```python
from build123d import *

# Parameters (mm, degrees)
SKETCH2_R           = 1.5
BOSS_EXTRUDE1_DEPTH = 2.54
SKETCH3_R           = 3.175
SKETCH3_R_2         = 1.5
BOSS_EXTRUDE2_DEPTH = 0.635
SKETCH4_W           = 6.35
SKETCH4_H           = 3
BOSS_EXTRUDE3_DEPTH = 3


with BuildPart() as part:
    # Sketch2 → Boss-Extrude1 (new body)
    with BuildSketch(Plane.XY):
        with BuildLine():
            Line((186.055, 33.49625), (189.23, 31.115))
            ThreePointArc((189.23, 31.115), (190.164806331, 29.994903166), (190.5, 28.575))
            Line((190.5, 28.575), (190.5, 0))
            Line((190.5, 0), (154.305, 0))
            Line((154.305, 0), (154.305, 29.44))
            ThreePointArc((154.305, 29.44), (154.676974388, 30.338025612), (155.575, 30.71))
            Line((155.575, 30.71), (161.925, 30.71))
            ThreePointArc((161.925, 30.71), (162.482139282, 30.58126939), (162.926332297, 30.221174521))
            Line((162.926332297, 30.221174521), (166.306150062, 25.888825479))
            ThreePointArc((166.306150062, 25.888825479), (166.750343077, 25.52873061), (167.307482358, 25.4))
            Line((167.307482358, 25.4), (175.563715168, 25.4))
            ThreePointArc((175.563715168, 25.4), (176.141475824, 25.539030228), (176.592738534, 25.925680906))
            Line((176.592738534, 25.925680906), (181.577441586, 32.817047734))
            ThreePointArc((181.577441586, 32.817047734), (183.673830399, 34.095340236), (186.055, 33.49625))
        make_face()
        with Locations((184.15, 30.95625)):
            Circle(SKETCH2_R, mode=Mode.SUBTRACT)
    extrude(amount=BOSS_EXTRUDE1_DEPTH)

    # Sketch3 → Boss-Extrude2 (add)
    with BuildSketch(Plane.XY.offset(2.54)):
        with Locations(Location((184.15, 30.95625, 0), (0, 0, 144.120815799))):
            Circle(SKETCH3_R)
        with Locations((184.15, 30.95625)):
            Circle(SKETCH3_R_2, mode=Mode.SUBTRACT)
    extrude(amount=BOSS_EXTRUDE2_DEPTH)

    # Sketch4 → Boss-Extrude3 (add)
    with BuildSketch(Plane(origin=(0, 0, 0), x_dir=(-1, 0, 0), z_dir=(0, 0, -1))):
        with Locations((-184.15, 27.94)):
            Rectangle(SKETCH4_W, SKETCH4_H)
        with Locations((-158.75, 27.94)):
            Rectangle(SKETCH4_W, SKETCH4_H)
    extrude(amount=BOSS_EXTRUDE3_DEPTH)

    # Mirror1: part across plane


with BuildPart() as part_1:
    add(part.part)
    add(part.part.mirror(Plane.ZX))


solid = part_1.part
```
Geometry: final body of the model. Coordinates: model frame, mm. A direction names the side the tool comes from. Round coordinates to 2 decimals unless told otherwise and drop trailing zeros. Order: outer loops, then holes, each group sorted by start corner. A loop starts at its lowest first (then second) coordinate and runs counter-clockwise, first axis right, second up. Notation, with made-up numbers: (8.5, 51) - (55.5, 51) arc R33 ccw to (55.5, 85) - close; hole circle Ø1 at (-32.5, 16). An arc over 180 degrees is marked (long way). Write item = value, one per line. Start each with the question number.
Q1. Pull-direction query (Y, two-part tool) for faces 4 (the flat face through (187.62, 32.322, 1.252)), 5 (the flat face through (184, 26.44, -1)), 6 (the flat face through (184, -28, -3)); classes: +Y half, -Y half, draft (parallel to the pull), parting line (faces both ways), or undercut.
Q2. Cut plane D-D on x = 171.5. Return the cut outline in (y, z).
Q3. Cut plane A-A on x = 184.15. Return the cut outline in (y, z) (3 decimals).
Q4. Cut plane B-B on z = -1. Return the cut outline in (x, y) (3 decimals).
Q5. Cut plane C-C on y = 5. Return the cut outline in (x, z) (3 decimals), and give its area (3 significant figures).
Q6. Access query for faces 1 (the flat face through (184, -29.44, -1)), 2 (the flat face through (161.925, 28, -1)), 3 (the flat face through (155.575, -28, -1)). Directions: +Z, -Z, +X, -X, +Y, -Y. A direction counts if a zero-diameter tool reaches every point of the face in a straight line with its end or side. Return the directions, or none.
Q7. Pin query (flat end, axial travel): pin 1 (11 mm diameter, centred on x = 168, y = 16, fed in from +Z); pin 2 (2.5 mm diameter, centred on x = 157.5, z = -2, fed in from -Y); pin 3 (1.3 mm diameter, centred on x = 157.5, z = 1.5, fed in from +Y); pin 4 (5 mm diameter, centred on x = 184.15, y = 30.96, fed in from -Z). Return the tip coordinate at first contact, or that it passes through.
Q8. Ray query, line 1 (Y direction, x = 184.15, z = 1.4); line 2 (Y direction, x = 184, z = 1.5); line 3 (Z direction, x = 158, y = 6). Return the intervals inside material, ascending. Write a range as from..to.
Outcome:
q1.face_4 = +Y half
q1.face_5 = undercut
q1.face_6 = draft
q2.outline = (-25.4, 0) - (25.4, 0) - (25.4, 2.54) - (-25.4, 2.54) - close
q3.outline = (-34.131, 0) - (-32.456, 0) - (-32.456, 3.175) - (-34.131, 3.175) - close; (-29.456, 0) - (-29.44, 0) - (-29.44, -3) - (-26.44, -3) - (-26.44, 0) - (26.44, 0) - (26.44, -3) - (29.44, -3) - (29.44, 0) - (29.456, 0) - (29.456, 3.175) - (27.781, 3.175) - (27.781, 2.54) - (-27.781, 2.54) - (-27.781, 3.175) - (-29.456, 3.175) - close; (32.456, 0) - (34.131, 0) - (34.131, 3.175) - (32.456, 3.175) - close
q4.outline = (155.575, -29.44) - (161.925, -29.44) - (161.925, -26.44) - (155.575, -26.44) - close; (155.575, 26.44) - (161.925, 26.44) - (161.925, 29.44) - (155.575, 29.44) - close; (180.975, -29.44) - (187.325, -29.44) - (187.325, -26.44) - (180.975, -26.44) - close; (180.975, 26.44) - (187.325, 26.44) - (187.325, 29.44) - (180.975, 29.44) - close
q5.outline = (154.305, 0) - (190.5, 0) - (190.5, 2.54) - (154.305, 2.54) - close
q5.area = 91.9 mm^2
q6.face_1 = -Z, +X, -X, -Y
q6.face_2 = -Z, +Y, -Y
q6.face_3 = -Z, -X, +Y, -Y
q7.pin_1 = 2.54
q7.pin_2 = -29.44
q7.pin_3 = 30.71
q7.pin_4 = -3
q8.line_1 = -34.13..-32.46, -29.46..29.46, 32.46..34.13
q8.line_2 = -34.13..-32.45, -29.46..29.46, 32.45..34.13
q8.line_3 = 0..2.54
